The drawing under review shows one solid part. Ordinate dimensions are in mm from its lowest x, y, z. A direction names the side the tool comes from. Coordinates: 2 decimals unless noted, no trailing zeros. Order: outer loops, then holes, each group sorted by start corner. A loop starts at its lowest first (then second) coordinate and runs counter-clockwise, first axis right, second up.
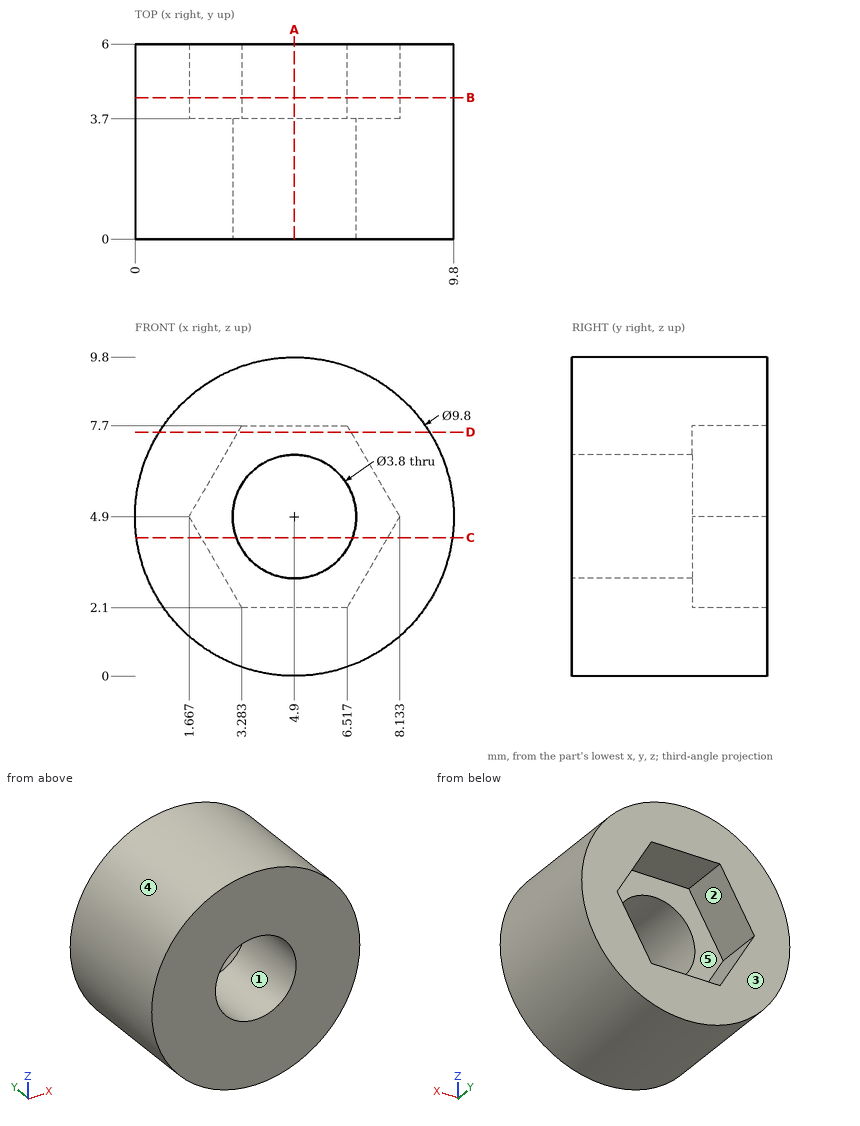
(1) Machinability: for the marked faces 1 and 2, which of the approach directions +Z, -Z, +X, -X, +Y, -Y give a long, thin tool a straight path to every point of the face, cutting with its end or side? Answer none if there is none.
A:
face 1: +Y, -Y
face 2: +Y
(2) For pin 1 Ø2 at (x, y) = (2, 5) entering from +Z; pin 2 Ø1 at (x, y) = (1.5, 4) entering from +Z; pin 3 Ø0.7 at (x, y) = (4, 5) entering from +Z, all flat-tipped, find the tip position at first contact; note any pin that passes through.
A:
pin 1: stops at z = 9.42
pin 2: stops at z = 8.85
pin 3: stops at z = 9.77
(3) Draft analysis for pull direction Z (two halves, no side actions). For the marked faces 3, 4 and 5, state which applies: released by +Z, released by -Z, zero draft, split by the parting line, or undercut.
A:
face 3: zero draft
face 4: split by the parting line
face 5: undercut
(4) We need section B-B, the plane y = 4.35. Write out the cut boundary in (x, z).
A:
outline: circle Ø9.8 at (4.9, 4.9); hole (1.67, 4.9) - (3.28, 2.1) - (6.52, 2.1) - (8.13, 4.9) - (6.52, 7.7) - (3.28, 7.7) - close
(5) We need section C-C, the plane z = 4.25. Write out the cut boundary in (x, y) (1 decimal).
A:
outline: (0, 0) - (3.1, 0) - (3.1, 3.7) - (2, 3.7) - (2, 6) - (0, 6) - close; (6.7, 0) - (9.8, 0) - (9.8, 6) - (7.8, 6) - (7.8, 3.7) - (6.7, 3.7) - close
(6) We need section D-D, the plane z = 7.5. Write out the cut boundary in (x, y).
A:
outline: (0.75, 0) - (9.05, 0) - (9.05, 6) - (6.63, 6) - (6.63, 3.7) - (3.17, 3.7) - (3.17, 6) - (0.75, 6) - close
(7) We need section A-A, the plane x = 4.9. Write out the cut boundary in (y, z).
A:
outline: (0, 0) - (6, 0) - (6, 2.1) - (3.7, 2.1) - (3.7, 3) - (0, 3) - close; (0, 6.8) - (3.7, 6.8) - (3.7, 7.7) - (6, 7.7) - (6, 9.8) - (0, 9.8) - close
(8) Wall thickness on probe 1 along Z at (x, y) = (4.9, 2.25); probe 2 along Y at (x, z) = (2.5, 5.75): over which ranges is each line inside the solid? List them lowest first.
A:
probe 1: z = 0 to 3, 6.8 to 9.8
probe 2: y = 0 to 3.7
